Here's the drawing with two shaded views (mm, measured from the low corner). I have some questions. Coordinates: 2 decimals unless noted, no trailing zeros. Order: outer loops, then holes, each group sorted by start corner. A loop starts at its lowest first (then second) coordinate and runs counter-clockwise, first axis right, second up. Notation, with made-up numbers: (39, 37.5) -> (80, 37.5) arc R18 ccw to (80, 41.5) -> close; hole circle Ø1 at (49.25, -18). An arc over 180 degrees is marked (long way). Write item = value, one per line.
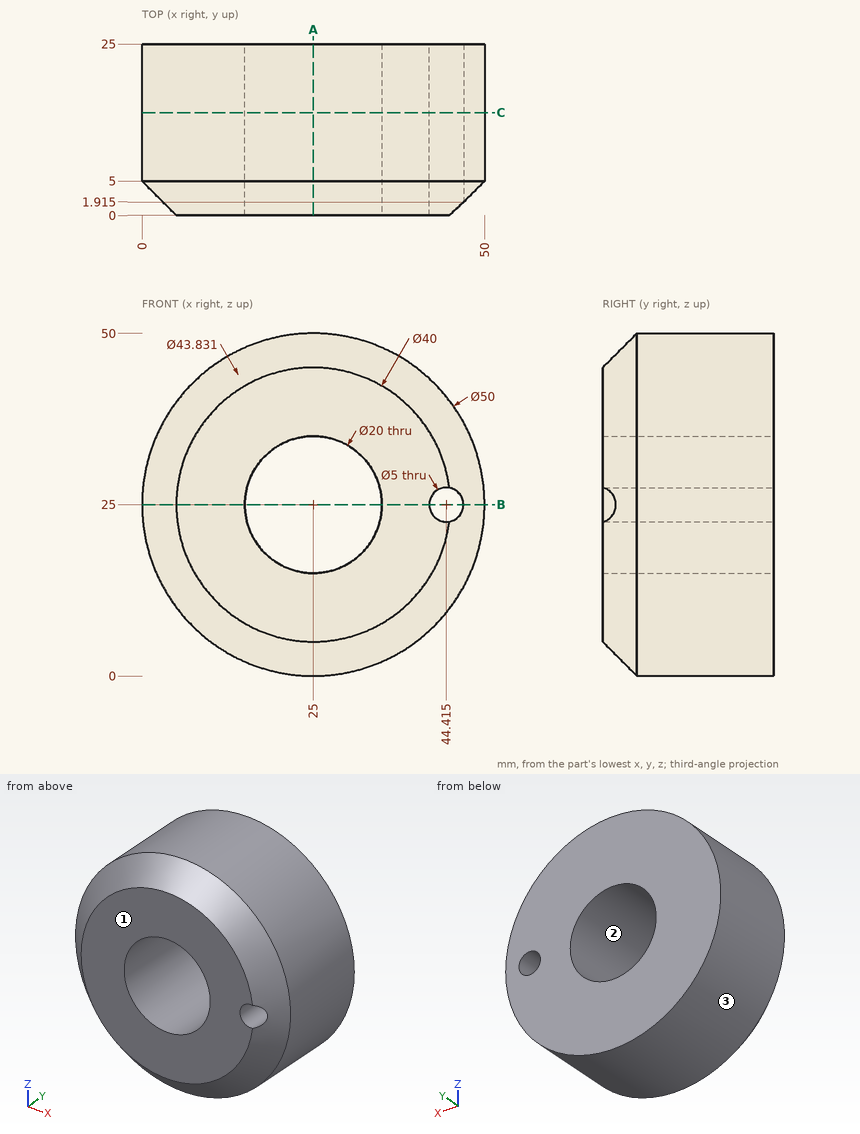
Item 1: I want a section at C-C, the plane y = 15. Please give me the cut outline in (x, z) (1 decimal).
A:
outline = circle Ø50 at (25, 25); hole circle Ø20 at (25, 25); hole circle Ø5 at (44.4, 25)
Item 2: I'm going to push flat-ended pins straight in: P1, Ø2, axis at x = 8, y = 19.5, coming from the +Z side; P2, Ø12, axis at x = 25, z = 25, coming from the -Y side; P3, Ø3, axis at x = 29, y = 19, coming from the -Z side (1 decimal); P4, Ø1.5, axis at x = 39, y = 9, coming from the +Z side. Where does each tip first touch, or does it pass through?
A:
P1 = 44.21
P2 = through
P3 = 0.1
P4 = 46.2
Item 3: I want a section at B-B, the plane z = 25. Please give me the cut outline in (x, y) (1 decimal), plus the area to 3 significant figures.
A:
outline = (0, 5) -> (5, 0) -> (15, 0) -> (15, 25) -> (0, 25) -> close; (35, 0) -> (41.9, 0) -> (41.9, 25) -> (35, 25) -> close; (46.9, 1.9) -> (50, 5) -> (50, 25) -> (46.9, 25) -> close
area = 602 mm2
Item 4: If I drill on probe 1 along Z at (x, y) = (25, 22); probe 2 along X at (y, z) = (7.5, 19); probe 3 along Z at (x, y) = (18, 1), over which ranges is the centre line in solid material (lowest first)?
A:
probe_1 = 0 to 15, 35 to 50
probe_2 = 0.73 to 17, 33 to 49.27
probe_3 = 5.2 to 17.86, 32.14 to 44.8
Item 5: If we mould it in two halves opening along X, with no side actions, what happens to the marked faces 1, 2 and 3? For each: pulls with the +X half, pulls with the -X half, needs draft (parallel to the pull), parting line crosses it, or undercut.
A:
face_1 = needs draft
face_2 = undercut
face_3 = parting line crosses it
Item 6: I want a section at A-A, the plane x = 25. Please give me the cut outline in (y, z).
A:
outline = (0, 5) -> (5, 0) -> (25, 0) -> (25, 15) -> (0, 15) -> close; (0, 35) -> (25, 35) -> (25, 50) -> (5, 50) -> (0, 45) -> close
